Verification items for the finished model (mm, model axes). A direction names the side the tool comes from. Coordinates: 2 decimals unless noted, no trailing zeros. Write each loop counter-clockwise with the first axis right and the second up, starting at its lowest first coordinate (ties: lowest second). Pieces come first, ordered by that corner, then holes. Notation, with made-up numbers: M -29,10.5 L -14,10.5 A20 ccw -14,43.5 Z; hole C -18,-18 d1. An arc over 180 degrees is marked long. One line per item, written item: value.
```python
from build123d import *

# Parameters (mm, degrees)
F0_W     = 88
F0_H     = 70
F1_DEPTH = 10
F2_W     = 32
F2_H     = 70
F3_DEPTH = 5
F2_R     = 2.5
F4_DEPTH = 10.001
F5_R     = 2
F6_DEPTH = 12


with BuildPart() as f1:
    # F0 (on Front) → F1 (new body)
    with BuildSketch(Plane.XZ):
        with Locations((-68.961055, 46.389333)):
            Rectangle(F0_W, F0_H)
    extrude(amount=F1_DEPTH)

    # F2 (on face) → F3 (cut)
    with BuildSketch(Plane.XZ.offset(10)):
        with Locations((-50.961055, 46.389333)):
            Rectangle(F2_W, F2_H)
    extrude(amount=-F3_DEPTH, mode=Mode.SUBTRACT)

    # F2 (on face) → F4 (cut, through all)
    with BuildSketch(Plane.XZ.offset(10)):
        with Locations((-102.961055, 70.389333)):
            Circle(F2_R)
        with Locations((-72.961055, 70.389333)):
            Circle(F2_R)
        with Locations((-102.961055, 22.389333)):
            Circle(F2_R)
        with Locations((-72.961055, 22.389333)):
            Circle(F2_R)
    extrude(amount=-F4_DEPTH, mode=Mode.SUBTRACT)

    # F5 (on face) → F6 (cut)
    with BuildSketch(Plane.YZ.offset(-24.961055)):
        with Locations((-5, 26.389333)):
            Circle(F5_R)
        with Locations((-5, 66.389333)):
            Circle(F5_R)
    extrude(amount=-F6_DEPTH, mode=Mode.SUBTRACT)


solid = f1.part
```
Item 1: Go/stop test with flat-tipped pins: P1, Ø2.5, axis at y = -5, z = 26.39, coming from the +X side; P2, Ø6.5, axis at x = -72.96, z = 22.39, coming from the +Y side; P3, Ø6, axis at x = -39, z = 67.5, coming from the -Y side. Record where each tip stops, or that it passes through.
The answers:
P1: stops at x = -36.96
P2: stops at y = 0
P3: stops at y = -5
Item 2: Scan lines: line 1 (Z direction, x = -73, y = -2); line 2 (X direction, y = -7.5, z = 54.5); line 3 (X direction, y = -7.5, z = 68.5). Record each from-to range of solid material in increasing order.
The answers:
line 1: z = 11.39 to 19.89, 24.89 to 67.89, 72.89 to 81.39
line 2: x = -112.96 to -66.96, -34.96 to -24.96
line 3: x = -112.96 to -104.6, -101.32 to -74.6, -71.32 to -66.96, -34.96 to -24.96
Item 3: Draft check along X on faces 4 (the face through (-70.577, -5.07, 71.14)), 5 (the face through (-30.877, -3.092, 66.99)), 6 (the face through (-36.961, -4, 26)). Enter one of: released by +X, released by -X, zero draft, split by the parting line, or undercut.
The answers:
face 4: undercut
face 5: zero draft
face 6: released by +X
Item 4: Cross-section at B-B, the plane z = 71.5. Enter the section's corners in (x, y), and give its area (3 significant figures).
The answers:
outline: M -112.96,-10 L -105.2,-10 L -105.2,0 L -112.96,0 Z; M -100.72,-10 L -75.2,-10 L -75.2,0 L -100.72,0 Z; M -70.72,-10 L -66.96,-10 L -66.96,-5 L -34.96,-5 L -34.96,-10 L -24.96,-10 L -24.96,0 L -70.72,0 Z
area: 630 mm²
Item 5: Cross-section at A-A, the plane y = -8.5. Enter the section's corners in (x, z), and give its area (3 significant figures).
The answers:
outline: M -112.96,11.39 L -66.96,11.39 L -66.96,81.39 L -112.96,81.39 Z; M -34.96,11.39 L -24.96,11.39 L -24.96,81.39 L -34.96,81.39 Z; hole C -102.96,22.39 d5; hole C -102.96,70.39 d5; hole C -72.96,22.39 d5; hole C -72.96,70.39 d5
area: 3,840 mm²
Item 6: Access from +Z, -Z, +X, -X, +Y, -Y to the whole of each face (thin tool, end or side, straight path). Record for faces 1 (the face through (-36.961, -4, 66)), 2 (the face through (-30.877, -3.092, 26.99)), 3 (the face through (-51, -5, 47)).
The answers:
face 1: +X, -Y
face 2: +X
face 3: +Z, -Z, -Y
Item 7: Cross-section at C-C, the plane z = 40. Enter the section's corners in (x, y).
The answers:
outline: M -112.96,-10 L -66.96,-10 L -66.96,-5 L -34.96,-5 L -34.96,-10 L -24.96,-10 L -24.96,0 L -112.96,0 Z
